Check sheet for the modelled part. Datum: model origin and axes. Units: mm. A direction names the side the tool comes from. Round coordinates to 2 decimals unless told otherwise and drop trailing zeros. Loops run counter-clockwise (first coordinate to the right, second up) from the corner with the lowest first, then second, coordinate; pieces in that order, holes last. Notation, with made-up numbers: (-35.75, 27) - (-19.75, 27) arc R20 ccw to (-19.75, 33) - close; hole circle Ø5 at (-35, 53). An arc over 180 degrees is marked (long way). Answer in a Markdown table with one row per item. Add a question column.
(1) Access from +Z, -Z, +X, -X, +Y, -Y to the whole of each face (thin tool, end or side, straight path). Record for faces 1 (the flat face through (41, -16, -3.175)), 2 (the flat face through (3, 0.254, -80)), 3 (the flat face through (42, -28.905, 11)), 4 (the cylindrical face through (20.22, -30.47, -96.81)), 5 (the flat face through (41, -28.905, -94)).
(2) Cross-section at B-B on x = 52.5. Enter the section's corners in (y, z) (3 decimals).
(3) Cross-section at A-A on y = -5. Enter the section's corners in (x, z) (3 decimals).
(4) Mould release check, pull along Z, two halves, no side actions. Record for faces 6 (the flat face through (42, -32.08, -92)), 7 (the cylindrical face through (20.224, -30.47, 7.965)), 8 (the flat face through (42, -11, -82.55)), 9 (the flat face through (41, -11, 0)): +Z half, -Z half, draft (parallel to the pull), parting line (faces both ways), or undercut.
(5) Cross-section at D-D on z = -22. Enter the section's corners in (x, y).
(6) Gauge pin test, flat ends, axial feed: pin 1 (8.5 mm diameter, centred on x = 61.91, z = -93.66, fed in from -Y); pin 2 (1.3 mm diameter, centred on x = 80, z = -79.5, fed in from +Y); pin 3 (8 mm diameter, centred on x = 60.5, z = -34, fed in from -Y); pin 4 (1.5 mm diameter, centred on x = 53, y = -20.5, fed in from +Z). Record the tip position at first contact, or that the pin passes through.
(7) Thickness scan on line 1 along Z through (x, y) = (21, -10.5) (3 decimals); line 2 along Y through (x, z) = (43, -41); line 3 along Z through (x, y) = (13, 1.5). Record the ranges inside material, lowest first.
(8) Cross-section at C-C on x = 61. Enter the section's corners in (y, z) (3 decimals), then the cut area to 3 significant figures.
Autodesk Inventor part; units mm, degrees
ref_plane "YZ Plane" through (0, 0, 0) normal (1, 0, 0) x (0, 1, 0)
ref_plane "XZ Plane" through (0, 0, 0) normal (0, 1, 0) x (-1, 0, 0)
ref_plane "XY Plane" through (0, 0, 0) normal (0, 0, 1) x (1, 0, 0)
sketch "Sketch1" plane through (0, 0, 0) normal (0, 1, 0) x (-1, 0, 0)
  line L0 (0, 0) -> (-82.55, 0)
  line L1 (-82.55, 0) -> (-82.55, -82.55)
  line L2 (-82.55, -82.55) -> (0, -82.55)
  line L3 (0, -82.55) -> (0, 0)
  dimension "d0" = 82.55
  dimension "d1" = 82.55
extrude "Extrusion1" add sketch "Sketch1" along normal blind 7.62
sketch "Sketch2" plane through (0, 0, 0) normal (0, -1, 0) x (1, 0, 0)
  line L0 (82.55, 0) -> (82.55, -82.55)
  line L1 (82.55, 0) -> (0, 0)
  line L2 (0, 0) -> (0, -3.175)
  line L3 (0, -3.175) -> (82.55, -3.175)
  line L4 (82.55, -3.175) -> (82.55, 0)
  line L5 (82.55, -82.55) -> (0, -82.55)
  line L6 (0, -82.55) -> (0, -79.375)
  line L7 (0, -79.375) -> (82.55, -79.375)
  line L8 (82.55, -79.375) -> (82.55, -82.55)
  dimension "d4" = 82.55
  dimension "d5" = 3.175
  dimension "d6" = 82.55
  dimension "d7" = 3.175
extrude "Extrusion2" add sketch "Sketch2" along normal blind 32.0802
sketch "Sketch3" plane through (0, 7.62, 0) normal (0, 1, 0) x (1, 0, 0)
  line L0 (0, 82.55) -> (82.55, 82.55) construction
  line L1 (0, 0) -> (82.55, 82.55) construction
  line L2 (82.55, 0) -> (0, 0) construction
  line L3 (0, 82.55) -> (82.55, 0) construction
  circle A0 centre (3.0661, 3.0077) radius 1.27
  circle A1 centre (3.0661, 79.5423) radius 1.27
  circle A2 centre (79.4839, 79.5423) radius 1.27
  circle A3 centre (79.4839, 3.0077) radius 1.27
  line L4 (3.0661, 3.0077) -> (79.4839, 79.5423) construction
  line L5 (3.0661, 79.5423) -> (79.4839, 3.0077) construction
  dimension "d14" = 2.54
  dimension "d15" = 2.54
  dimension "d16" = 2.54
  dimension "d17" = 2.54
extrude "Extrusion3" cut sketch "Sketch3" against normal blind 7.366
sketch "Sketch4" plane through (82.55, 7.62, -82.55) normal (0, 0, -1) x (-1, 0, 0)
  line L0 (0, 0) -> (0, -39.7002)
  line L1 (0, -39.7002) -> (82.55, -39.7002)
  line L2 (82.55, -39.7002) -> (82.55, -36.5252)
  line L3 (82.55, -36.5252) -> (0, -36.5252)
  line L4 (0, -36.5252) -> (0, -39.7002)
  point P0 (82.55, -7.62)
  dimension "d20" = 82.55
  dimension "d21" = 3.175
extrude "Extrusion4" add sketch "Sketch4" along normal blind 22.225
sketch "Sketch5" plane through (0, 7.62, 0) normal (0, 0, 1) x (1, 0, 0)
  line L0 (82.55, -39.7002) -> (0, -39.7002)
  line L1 (0, -39.7002) -> (82.55, -39.7002)
  line L2 (82.55, -39.7002) -> (82.55, -36.5252)
  line L3 (82.55, -36.5252) -> (0, -36.5252)
  line L4 (0, -36.5252) -> (0, -39.7002)
  point P0 (0, -7.62)
  dimension "d24" = 82.55
  dimension "d25" = 3.175
extrude "Extrusion5" add sketch "Sketch5" along normal blind 22.225
sketch "Sketch6" plane through (0, -28.9052, 0) normal (0, 1, 0) x (1, 0, 0)
  line L0 (0, 0) -> (0, -22.225) construction
  line L1 (0, -22.225) -> (0, -11.1125) construction
  line L2 (0, -11.1125) -> (20.6375, -11.1125) construction
  line L3 (20.6375, -11.1125) -> (61.9125, -11.1125) construction
  line L4 (0, 79.375) -> (0, 104.775) construction
  line L5 (0, 104.775) -> (0, 93.6625) construction
  line L6 (0, 93.6625) -> (20.6375, 93.6625) construction
  line L7 (20.6375, 93.6625) -> (61.9125, 93.6625) construction
  circle A0 centre (20.6375, -11.1125) radius 3.175
  circle A1 centre (20.6375, 93.6625) radius 3.175
  circle A2 centre (61.9125, 93.6625) radius 3.175
  circle A3 centre (61.9125, -11.1125) radius 3.175
  dimension "d28" = 11.1125
  dimension "d29" = 20.6375
  dimension "d30" = 41.275
  dimension "d31" = 11.1125
  dimension "d32" = 20.6375
  dimension "d33" = 90
  dimension "d34" = 41.275
  dimension "d35" = 180
  dimension "d36" = 6.35
  dimension "d37" = 6.35
  dimension "d38" = 6.35
  dimension "d39" = 6.35
extrude "Extrusion6" cut sketch "Sketch6" against normal blind 3.175
properties part number "TurntableBase2"
Answers:
| question | item | result |
|---|---|---|
| 1 | face 1 | +X, -X, -Y |
| 1 | face 2 | +Y |
| 1 | face 3 | +Z, +X, -X, +Y |
| 1 | face 4 | +Y, -Y |
| 1 | face 5 | -Z, +X, -X, +Y |
| 2 | outline | (-32.08, -104.775) - (-28.905, -104.775) - (-28.905, -82.55) - (7.62, -82.55) - (7.62, 0) - (-28.905, 0) - (-28.905, 22.225) - (-32.08, 22.225) - (-32.08, -3.175) - (0, -3.175) - (0, -79.375) - (-32.08, -79.375) - close |
| 3 | outline | (0, -82.55) - (82.55, -82.55) - (82.55, -79.375) - (0, -79.375) - close; (0, -3.175) - (82.55, -3.175) - (82.55, 0) - (0, 0) - close |
| 4 | face 6 | draft |
| 4 | face 7 | undercut |
| 4 | face 8 | -Z half |
| 4 | face 9 | +Z half |
| 5 | outline | (0, 0) - (82.55, 0) - (82.55, 7.62) - (0, 7.62) - close |
| 6 | pin 1 | stops at y = -32.08 |
| 6 | pin 2 | stops at y = 0.25 |
| 6 | pin 3 | stops at y = 0 |
| 6 | pin 4 | stops at z = 0 |
| 7 | line 1 | z = -82.55 to -79.375, -3.175 to 0 |
| 7 | line 2 | y = 0 to 7.62 |
| 7 | line 3 | z = -82.55 to 0 |
| 8 | outline | (-32.08, -104.775) - (-28.905, -104.775) - (-28.905, -96.704) - (-32.08, -96.704) - close; (-32.08, -90.621) - (-28.905, -90.621) - (-28.905, -82.55) - (7.62, -82.55) - (7.62, 0) - (-28.905, 0) - (-28.905, 8.071) - (-32.08, 8.071) - (-32.08, -3.175) - (0, -3.175) - (0, -79.375) - (-32.08, -79.375) - close; (-32.08, 14.154) - (-28.905, 14.154) - (-28.905, 22.225) - (-32.08, 22.225) - close |
| 8 | area | 935 mm^2 |
